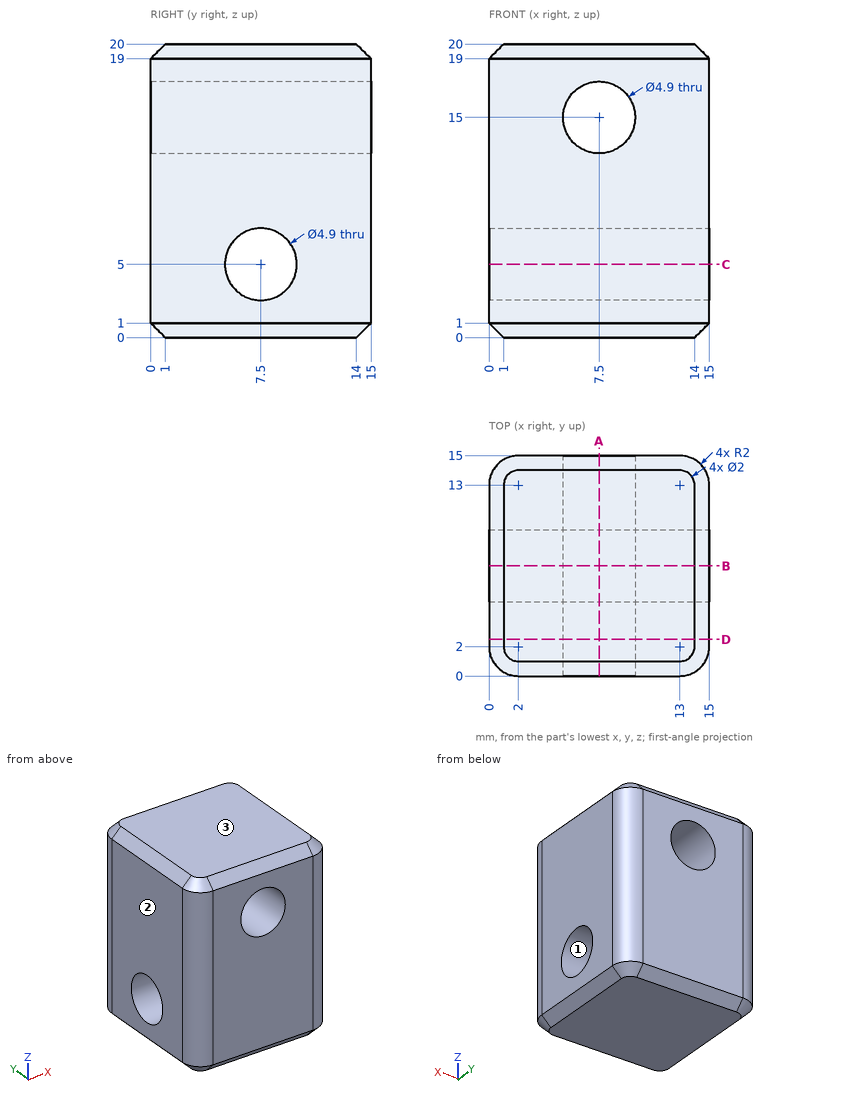
Geometry: see drawing. Coordinates: mm, zero at the bounding-box minimum. Round coordinates to 2 decimals unless told otherwise and drop trailing zeros. Loops run counter-clockwise (first coordinate to the right, second up) from the corner with the lowest first, then second, coordinate; pieces in that order, holes last. Notation, with made-up numbers: (-13.75, 17) -> (16.25, 17) arc R6 cw to (16.25, 24) -> close; hole circle Ø7 at (-9, 33). An arc over 180 degrees is marked (long way). Write each question's results on one line, items separated by ' | '.
Item 1: Cut plane C-C on z = 5. Return the cut outline in (x, y), and give its area (3 significant figures).
Answers below:
outline: (0, 2) arc R2 ccw to (2, 0) -> (13, 0) arc R2 ccw to (15, 2) -> (15, 5.05) -> (0, 5.05) -> close; (0, 9.95) -> (15, 9.95) -> (15, 13) arc R2 ccw to (13, 15) -> (2, 15) arc R2 ccw to (0, 13) -> close | area: 148 mm²
Item 2: Pin query (flat end, axial travel): pin 1 Ø4 at (y, z) = (7.5, 5) entering from +X. Return the tip coordinate at first contact, or that it passes through.
Answers below:
pin 1: passes through
Item 3: Line query: probe 1 along X at (y, z) = (4, 15); probe 2 along Z at (x, y) = (7.5, 9.25); probe 3 along Z at (x, y) = (7.5, 8.5). Output: solid intervals per line, ascending. Write a range as [from, to].
Answers below:
probe 1: x = [0, 5.05], [9.95, 15] | probe 2: z = [0, 3.29], [6.71, 12.55], [17.45, 20] | probe 3: z = [0, 2.76], [7.24, 12.55], [17.45, 20]
Item 4: Cut plane B-B on y = 7.5. Return the cut outline in (x, z), and give its area (3 significant figures).
Answers below:
outline: (0, 1) -> (1, 0) -> (14, 0) -> (15, 1) -> (15, 2.55) -> (0, 2.55) -> close; (0, 7.45) -> (15, 7.45) -> (15, 19) -> (14, 20) -> (1, 20) -> (0, 19) -> close; hole circle Ø4.9 at (7.5, 15) | area: 206 mm²
Item 5: Pull-direction query (Z, two-part tool) for the marked faces 1, 2 and 3; classes: pulls with the +Z half, pulls with the -Z half, needs draft (parallel to the pull), parting line crosses it, or undercut.
Answers below:
face 1: undercut | face 2: needs draft | face 3: pulls with the +Z half
Item 6: Cut plane A-A on x = 7.5. Return the cut outline in (y, z), and give its area (3 significant figures).
Answers below:
outline: (0, 1) -> (1, 0) -> (14, 0) -> (15, 1) -> (15, 12.55) -> (0, 12.55) -> close; (0, 17.45) -> (15, 17.45) -> (15, 19) -> (14, 20) -> (1, 20) -> (0, 19) -> close; hole circle Ø4.9 at (7.5, 5) | area: 206 mm²
Item 7: Cut plane D-D on y = 2.5. Return the cut outline in (x, z).
Answers below:
outline: (0, 1) -> (1, 0) -> (14, 0) -> (15, 1) -> (15, 19) -> (14, 20) -> (1, 20) -> (0, 19) -> close; hole circle Ø4.9 at (7.5, 15)
